from build123d import *
from build123d.topology import SkipClean

# Parameters (mm, degrees)
SKETCH1_W                   = 155
SKETCH1_H                   = 16
CUT_EXTRUDE1_DEPTH          = 81.735679845
CUT_EXTRUDE1_DEPTH_BACK     = 81.735679845
SKETCH2_R                   = 6.25
SKETCH4_W                   = 50
SKETCH4_H                   = 7
CUT_EXTRUDE3_DEPTH          = 38
BOSS_EXTRUDE1_DEPTH         = 5
SKETCH24_R                  = 12.875
CUT_EXTRUDE12_DEPTH         = 22
SKETCH12_R                  = 16
SKETCH12_R_2                = 10
CUT_EXTRUDE6_DEPTH          = 35
SKETCH13_R                  = 6
BOSS_EXTRUDE2_DEPTH         = 15
CHAMFER2_SIZE               = 0.5
SKETCH17_R                  = 16
SKETCH17_R_2                = 12.5
CUT_EXTRUDE9_DEPTH          = 75
SKETCH14_W                  = 1
SKETCH14_H                  = 1
BOSS_EXTRUDE3_DEPTH         = 35
CIRPATTERN1_COUNT           = 32
CUT_EXTRUDE10_DEPTH         = 96.227359548
CUT_EXTRUDE10_DEPTH_BACK    = 96.227359548
SKETCH20_W                  = 129.677908588
SKETCH20_H                  = 32
BOSS_EXTRUDE4_START         = 30
SKETCH22_R                  = 16
BOSS_EXTRUDE4_DEPTH         = 30
M10X1_25_TAPPED_HOLE1_D     = 8.8
M10X1_25_TAPPED_HOLE1_DEPTH = 30
M10X1_25_TAPPED_HOLE1_TIP   = 2.643786724


with BuildPart() as part:
    # Sketch1 → Revolve1 (revolve)
    with BuildSketch(Plane(origin=(0, 0, 0), x_dir=(1, 0, 0), z_dir=(0, 1, 0))):
        with Locations((0, -8)):
            Rectangle(SKETCH1_W, SKETCH1_H)
    revolve(axis=Axis((-77.5, 0, 0), (1, 0, 0)))

    # Sketch2 → Cut-Extrude1 (cut, two sides: drawn at the far end of the back side and taken through both)
    with BuildSketch(Plane(origin=(0, 0, 0), x_dir=(1, 0, 0), z_dir=(0, 1, 0)).offset(-CUT_EXTRUDE1_DEPTH_BACK)):
        with Locations(Location((-53.5, 0, 0), (0, 0, 270))):
            Circle(SKETCH2_R)
    extrude(amount=CUT_EXTRUDE1_DEPTH + CUT_EXTRUDE1_DEPTH_BACK, mode=Mode.SUBTRACT)

    # Sketch4 → Cut-Extrude3 (cut)
    with BuildSketch(Plane.ZY.offset(77.5)):
        Rectangle(SKETCH4_W, SKETCH4_H)
    extrude(amount=-CUT_EXTRUDE3_DEPTH, mode=Mode.SUBTRACT)

    # Sketch6 → Boss-Extrude1 (add)
    with BuildSketch(Plane.ZY.offset(77.5)):
        with BuildLine():
            Line((-15.612494996, 3.5), (15.612494996, 3.5))
            ThreePointArc((15.612494996, 3.5), (0, 16), (-15.612494996, 3.5))
        make_face()
        with BuildLine():
            Line((15.612494996, -3.5), (-15.612494996, -3.5))
            ThreePointArc((-15.612494996, -3.5), (0, -16), (15.612494996, -3.5))
        make_face()
    extrude(amount=BOSS_EXTRUDE1_DEPTH)

    # Sketch24 → Cut-Extrude12 (cut)
    with BuildSketch(Plane.ZY.offset(82.5)):
        Circle(SKETCH24_R)
    extrude(amount=-CUT_EXTRUDE12_DEPTH, mode=Mode.SUBTRACT)

    # Sketch12 → Cut-Extrude6 (cut)
    with BuildSketch(Plane(origin=(77.5, 0, 0), x_dir=(0, 0, -1), z_dir=(1, 0, 0))):
        with Locations(Location((0, 0, 0), (0, 0, 167.364374907))):
            Circle(SKETCH12_R)
        Circle(SKETCH12_R_2, mode=Mode.SUBTRACT)
    extrude(amount=-CUT_EXTRUDE6_DEPTH, mode=Mode.SUBTRACT)

    # Sketch13 → Boss-Extrude2 (add)
    with BuildSketch(Plane(origin=(77.5, 0, 0), x_dir=(0, 0, -1), z_dir=(1, 0, 0))):
        Circle(SKETCH13_R)
    extrude(amount=BOSS_EXTRUDE2_DEPTH)

    # Chamfer2
    chamfer2_edges = [part.edges().sort_by_distance(p)[0] for p in [
        (92.5, 0, 6),
    ]]
    chamfer(chamfer2_edges, length=CHAMFER2_SIZE)

    # Sketch17 → Cut-Extrude9 (cut)
    with BuildSketch(Plane(origin=(47.5, 0, 0), x_dir=(0, 0, -1), z_dir=(1, 0, 0))):
        with Locations(Location((0, 0, 0), (0, 0, 167.364374907))):
            Circle(SKETCH17_R)
        Circle(SKETCH17_R_2, mode=Mode.SUBTRACT)
    extrude(amount=-CUT_EXTRUDE9_DEPTH, mode=Mode.SUBTRACT)

    # Sketch14 → Boss-Extrude3 (add)
    with SkipClean():  # the faces are left unmerged after this step: merging them gives an invalid solid
        with BuildSketch(Plane(origin=(77.5, 0, 0), x_dir=(0, 0, -1), z_dir=(1, 0, 0))):
            with Locations((0, 10)):
                Rectangle(SKETCH14_W, SKETCH14_H)
        boss_extrude3 = extrude(amount=-BOSS_EXTRUDE3_DEPTH)

    # CirPattern1: Boss-Extrude3 ×32 about axis
    with SkipClean():  # the faces are left unmerged after this step: merging them gives an invalid solid
        cirpattern1_axis = Axis((0, 0, 0), (1, 0, 0))
        for i in range(1, CIRPATTERN1_COUNT):
            add(boss_extrude3.rotate(cirpattern1_axis, i * 360 / CIRPATTERN1_COUNT))

    # Sketch20 → Cut-Extrude10 (cut, two sides: drawn at the far end of the back side and taken through both)
    with BuildSketch(Plane(origin=(0, 0, 0), x_dir=(1, 0, 0), z_dir=(0, 1, 0)).offset(-CUT_EXTRUDE10_DEPTH_BACK)):
        with Locations((37.338954294, 0)):
            Rectangle(SKETCH20_W, SKETCH20_H)
    extrude(amount=CUT_EXTRUDE10_DEPTH + CUT_EXTRUDE10_DEPTH_BACK, mode=Mode.SUBTRACT)

    # Sketch22 → Boss-Extrude4 (add)
    with SkipClean():  # the faces are left unmerged after this step: merging them gives an invalid solid
        with BuildSketch(Plane(origin=(-27.5, 0, 0), x_dir=(0, 0, -1), z_dir=(1, 0, 0)).offset(BOSS_EXTRUDE4_START)):
            with Locations(Location((0, 0, 0), (0, 0, 167.364374907))):
                Circle(SKETCH22_R)
        extrude(amount=-BOSS_EXTRUDE4_DEPTH)

    # M10x1.25 Tapped Hole1
    with Locations(Plane(origin=(2.5, 0, 0), x_dir=(0, 0, -1), z_dir=(1, 0, 0))):
        with Locations((0, 0)):
            Hole(M10X1_25_TAPPED_HOLE1_D / 2, depth=M10X1_25_TAPPED_HOLE1_DEPTH)
            with Locations((0, 0, -(M10X1_25_TAPPED_HOLE1_DEPTH + M10X1_25_TAPPED_HOLE1_TIP / 2))):  # 118° drill point
                Cone(0, M10X1_25_TAPPED_HOLE1_D / 2, M10X1_25_TAPPED_HOLE1_TIP, mode=Mode.SUBTRACT)


solid = part.part
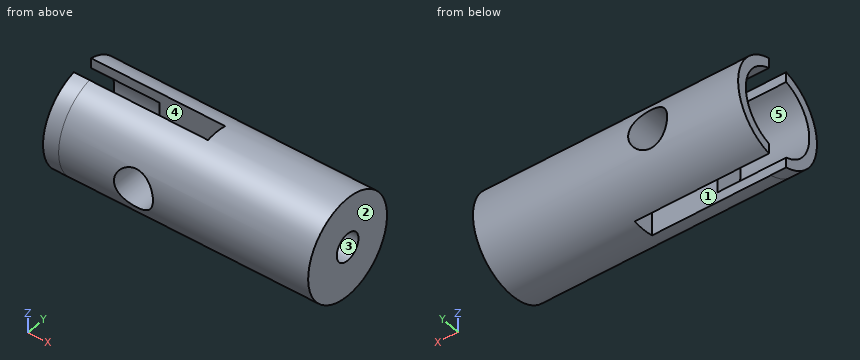
Build history of the part. All positions in model axes, mm. Face numbers are marked on the shaded views. A direction names the side the tool comes from. Give positions to 0.01 mm unless a question says otherwise; leave off trailing zeros. Order: outer loops, then holes, each group sorted by start corner. A loop starts at its lowest first (then second) coordinate and runs counter-clockwise, first axis right, second up. Notation, with made-up numbers: M 82,72.5 L 140,72.5 A22 cw 140,99.5 Z; hole C -24.5,-31 d8. An arc over 180 degrees is marked long. Use one line per item in the form item = value.
Q1. Which spindle directions (+Z, -Z, +X, -X, +Y, -Y) get a long thin tool onto all of the face, cutting with end or side? Do the marked faces 3, 4 and 5. Say none if no direction does.
Conclusion:
face_3 = +X
face_4 = +Z, -Z, -X
face_5 = -X
Q2. Slice it at D-D, the plane y = 8. Write the cut outline in (x, z).
Conclusion:
outline = M -82.5,-13.86 L 2.5,-13.86 L 2.5,13.86 L -82.5,13.86 L -82.5,10.09 L -60.5,10.09 L -60.5,-10.09 L -82.5,-10.09 Z; hole C -53.5,0 d12.5
Q3. Slice it at B-B, the plane x = -53.5. Write the cut outline in (y, z), and give its area (3 significant figures).
Conclusion:
outline = M -14.73,-6.25 A16 ccw -3.5,-15.61 L -3.5,-6.25 Z; M -14.73,6.25 L -3.5,6.25 L -3.5,15.61 A16 ccw Z; M 3.5,-15.61 A16 ccw 14.73,-6.25 L 3.5,-6.25 Z; M 3.5,6.25 L 14.73,6.25 A16 ccw 3.5,15.61 Z
area = 280 mm2
Q4. Pin check, flat tips, straight feed: P1, Ø1.5, axis at x = -32.5, y = 5, coming from the -Z side; P2, Ø7.5, axis at y = 0, z = 4, coming from the -X side; P3, Ø3, axis at x = -61.5, z = -10.5, coming from the +Y side; P4, Ø11, axis at x = -53.5, z = 0, coming from the +Y side. Stop position of each tip, or through.
Conclusion:
P1 = -15.43
P2 = -60.5
P3 = 13.23
P4 = through
Q5. Slice it at C-C, the plane z = 11.5. Write the cut outline in (x, y), and give its area (3 significant figures).
Conclusion:
outline = M -82.5,-11.12 L 2.5,-11.12 L 2.5,11.12 L -82.5,11.12 L -82.5,5.79 L -60.5,5.79 L -60.5,3.5 L -39.5,3.5 L -39.5,-3.5 L -60.5,-3.5 L -60.5,-5.79 L -82.5,-5.79 Z
area = 1,490 mm2
Q6. Pull direction Y, two halves, no side cores. Call the marked faces 1 and 2: released by +Y, released by -Y, zero draft, split by the parting line, or undercut.
Conclusion:
face_1 = undercut
face_2 = zero draft
Q7. Wall check: probe 1 along X at (y, z) = (-10, 0); probe 2 along Y at (x, z) = (-27, 0). Give the ranges that are in metal, low to high.
Conclusion:
probe_1 = -60.5 to -59.75, -47.25 to 2.5
probe_2 = -16 to -4.4, 4.4 to 16
